from build123d import *

# Parameters (mm, degrees)
SKETCH_1_W                 = 5
SKETCH_1_H                 = 60
EXTRUDE_1_DEPTH            = 60
SKETCH_2_R                 = 5
SKETCH_4_R                 = 3.5
CUT_EXTRUDE_1_DEPTH        = 137.839321834
HOLE_WIZARD_M81_AT_2_COUNT = 2
HOLE_WIZARD_M81_AT_2_PITCH = 29.154759474
CUT_EXTRUDE_2_DEPTH        = 89.600225733
CUT_EXTRUDE_2_DEPTH_BACK   = 89.600225733
SKETCH_7_W                 = 23
SKETCH_7_H                 = 11
SKETCH_7_W_2               = 22


with BuildPart() as part:
    # Эскиз1 → Вытянуть-Тонкостенный1 (new, symmetric)
    with BuildSketch(Plane.XY):
        with Locations((2.5, 30)):
            Rectangle(SKETCH_1_W, SKETCH_1_H)
    extrude(amount=EXTRUDE_1_DEPTH, both=True)

    # По траектории1: sweep along a curve in space
    with BuildLine() as sweep_1_path:
        Line((5, 60, 60), (5, 60, -60))
    # Эскиз2 → По траектории1 (sweep)
    with BuildSketch(Plane.XY.offset(60)):
        with Locations((5, 60)):
            Circle(SKETCH_2_R)
    sweep(path=sweep_1_path.line)

    # Эскиз4 → Вырез-Вытянуть1 (cut, through all)
    with BuildSketch(Plane.XY.offset(60)):
        with Locations((5, 60)):
            Circle(SKETCH_4_R)
    extrude(amount=-CUT_EXTRUDE_1_DEPTH, mode=Mode.SUBTRACT)

    # Эскиз5 → Зенковка для  винта с плоской головкой M81 (revolve, cut)
    with BuildSketch(Plane(origin=(5, 30, 45), x_dir=(0, 0, -1), z_dir=(0, 1, 0))):
        Polygon((0, 0), (0, 5), (4.5, 5), (4.5, 4.15), (8.65, 0), align=None)
    hole_wizard_m81 = revolve(axis=Axis((11.35, 30, 45), (-1, 0, 0)), mode=Mode.SUBTRACT)

    # Зенковка для  винта с плоской головкой M81 at 2: Зенковка для  винта с плоской головкой M81 ×2
    with Locations(*[Vector(0, -0.5144957554275265, -0.8574929257125442) * (i * HOLE_WIZARD_M81_AT_2_PITCH) for i in range(1, HOLE_WIZARD_M81_AT_2_COUNT)]):
        add(hole_wizard_m81, mode=Mode.SUBTRACT)

    # Зеркальное отражение1: Зенковка для  винта с плоской головкой M81 across plane
    add(hole_wizard_m81.mirror(Plane.XY), mode=Mode.SUBTRACT)

    # Зеркальное отражение1 copy 1 sketch → Зеркальное отражение1 copy 1 (revolve, cut)
    with BuildSketch(Plane(origin=(5, 15, -20), x_dir=(0, 0, 1), z_dir=(0, 1, 0))):
        Polygon((0, 0), (0, -5), (4.5, -5), (4.5, -4.15), (8.65, 0), align=None)
    revolve(axis=Axis((11.35, 15, -20), (1, 0, 0)), mode=Mode.SUBTRACT)

    # Эскиз7 → Вырез-Вытянуть2 (cut, two sides: drawn at the far end of the back side and taken through both)
    with BuildSketch(Plane(origin=(5, 0, 0), x_dir=(0, 0, -1), z_dir=(1, 0, 0)).offset(-CUT_EXTRUDE_2_DEPTH_BACK)):
        with Locations((48.5, 59.5)):
            Rectangle(SKETCH_7_W, SKETCH_7_H)
        with Locations((-48.5, 59.5)):
            Rectangle(SKETCH_7_W, SKETCH_7_H)
        with Locations((0, 59.5)):
            Rectangle(SKETCH_7_W_2, SKETCH_7_H)
    extrude(amount=CUT_EXTRUDE_2_DEPTH + CUT_EXTRUDE_2_DEPTH_BACK, mode=Mode.SUBTRACT)


solid = part.part
The model under review builds one solid part; all positions refer to its coordinate system, in mm. A direction names the side the tool comes from. Round coordinates to 2 decimals unless told otherwise and drop trailing zeros. Order: outer loops, then holes, each group sorted by start corner. A loop starts at its lowest first (then second) coordinate and runs counter-clockwise, first axis right, second up. Notation, with made-up numbers: (-37, -5) -> (-7, -5) arc R26 ccw to (-7, 19) -> close; hole circle Ø11 at (74, 0). An arc over 180 degrees is marked (long way). Write item = value, one per line. Start each with the question number.
Item 1: Consider section C-C on y = 41. Write out the cut boundary in (x, z), plus the area to 3 significant figures.
Item 2: Consider section D-D on z = -6.5. Write out the cut boundary in (x, y).
Item 3: Consider section B-B on z = 45. Write out the cut boundary in (x, y), plus the area to 3 significant figures.
Item 4: Consider section A-A on y = 30. Write out the cut boundary in (x, z), plus the area to 3 significant figures.
Item 5: Clearance check with flat-ended pins moving along their axes: pin 1 Ø14.5 at (y, z) = (15, -20) entering from +X; pin 2 Ø4 at (x, y) = (5, 60) entering from +Z; pin 3 Ø5.5 at (x, z) = (1.5, -50) entering from +Y; pin 4 Ø12 at (y, z) = (22.5, -5.5) entering from +X. State where each tip first meets the part, or that it passes through.
Item 6: For line 1 along Z through (x, y) = (0.65, 30); line 2 along Z through (x, y) = (9.25, 59.5); line 3 along Y through (x, z) = (5.25, -24), list the stretches that pass through material, from the lowest coordinate up.
Item 7: For faces 1 (the face through (2, 54, 49)), 2 (the face through (2.7, 57, -11)), 3 (the face through (2.7, 57, -37)), 4 (the face through (5, 27, 1)), list the 3-axis set-ups (+Z, -Z, +X, -X, +Y, -Y) from which the entire face can be reached by the end or side of a thin tool; tool diameter is ignored.
Item 8: Mouldability with a two-part tool opening along Z and no side actions: class faces 5 (the face through (1.11, 28.57, -40.46)), 6 (the face through (2, 27, 60)), 7 (the face through (2, 0, 1)) as released by +Z, released by -Z, zero draft, split by the parting line, or undercut.
Conclusion:
q1.outline = (0, -60) -> (5, -60) -> (5, 60) -> (0, 60) -> close
q1.area = 600 mm2
q2.outline = (0, 0) -> (5, 0) -> (5, 54) -> (0, 54) -> close
q3.outline = (0, 0) -> (5, 0) -> (5, 21.35) -> (0.85, 25.5) -> (0, 25.5) -> close; (0, 34.5) -> (0.85, 34.5) -> (5, 38.65) -> (5, 54) -> (0, 54) -> close
q3.area = 208 mm2
q4.outline = (0, -60) -> (5, -60) -> (5, -53.65) -> (0.85, -49.5) -> (0, -49.5) -> close; (0, -40.5) -> (0.85, -40.5) -> (5, -36.35) -> (5, 36.35) -> (0.85, 40.5) -> (0, 40.5) -> close; (0, 49.5) -> (0.85, 49.5) -> (5, 53.65) -> (5, 60) -> (0, 60) -> close
q4.area = 476 mm2
q5.pin_1 = 3.6
q5.pin_2 = through
q5.pin_3 = 54
q5.pin_4 = 5
q6.line_1 = -60 to -49.5, -40.5 to 40.5, 49.5 to 60
q6.line_2 = -37 to -11, 11 to 37
q6.line_3 = 55.01 to 56.51, 63.49 to 64.99
q7.face_1 = +Z, +X, -X, +Y
q7.face_2 = +X, -X, +Y
q7.face_3 = -Z, +X, -X, +Y
q7.face_4 = +Z, -Z, +X, -Y
q8.face_5 = undercut
q8.face_6 = released by +Z
q8.face_7 = zero draft
